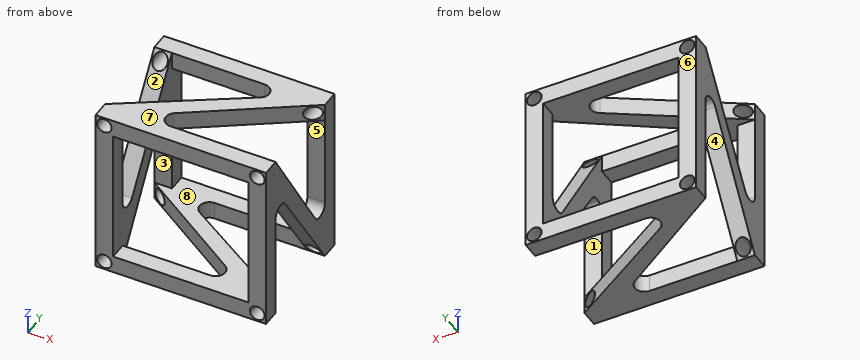
Autodesk Inventor part; units mm, degrees
ref_plane "YZ Plane" through (0, 0, 0) normal (1, 0, 0) x (0, 1, 0)
ref_plane "XZ Plane" through (0, 0, 0) normal (0, 1, 0) x (-1, 0, 0)
ref_plane "XY Plane" through (0, 0, 0) normal (0, 0, 1) x (1, 0, 0)
sketch "Sketch1" plane through (0, 0, 0) normal (0, 1, 0) x (-1, 0, 0)
  line L0 (0, 0) -> (35, 0)
  line L1 (35, 0) -> (35, 35)
  line L2 (35, 35) -> (0, 35)
  line L3 (0, 35) -> (0, 0)
  line L4 (3.6, 3.6) -> (31.4, 3.6)
  line L5 (31.4, 3.6) -> (31.4, 31.4)
  line L6 (31.4, 31.4) -> (3.6, 31.4)
  line L7 (3.6, 31.4) -> (3.6, 3.6)
  circle A0 centre (33.2, 33.2) radius 1.5
  circle A1 centre (33.2, 1.8) radius 1.5
  circle A2 centre (1.8, 1.8) radius 1.5
  circle A3 centre (1.8, 33.2) radius 1.5
  dimension "d0" = 35
  dimension "d1" = 35
  dimension "d2" = 3.6
  dimension "d3" = 3.6
  dimension "d4" = 3.6
  dimension "d5" = 3.6
  dimension "d6" = 3
  dimension "d7" = 1.8
  dimension "d8" = 1.8
  dimension "d9" = 3
  dimension "d10" = 1.8
  dimension "d11" = 1.8
  dimension "d12" = 3
  dimension "d13" = 1.8
  dimension "d14" = 1.8
  dimension "d15" = 3
  dimension "d16" = 1.8
  dimension "d17" = 1.8
extrude "Extrusion1" add sketch "Sketch1" along normal blind 25.9
sketch "Sketch3" plane through (-35, 0, 35) normal (0, 0, 1) x (1, 0, 0)
  line L0 (0, 25.9) -> (35, 25.9)
  line L1 (0, 0) -> (35, 0)
  line L2 (0, 0) -> (0, 25.9)
  line L3 (18.01, 21.1181) -> (18.01, 21.1181)
  line L4 (0, 0) -> (0, 25.9)
  line L5 (31.4, 0) -> (31.4, 25.9)
  line L6 (31.4, 3.6) -> (13.39, 3.6)
  arc A0 (12.1285, 7.1519) -> (13.39, 3.6) centre (13.39, 5.6) ccw
  line L7 (3.6, 22.3) -> (22.6522, 22.3)
  line L8 (3.6, 22.3) -> (0, 22.3)
  line L9 (31.4, 3.6) -> (31.4, 0)
  line L10 (0, 22.3) -> (0, 25.9)
  line L11 (31.4, 22.2467) -> (31.4, 25.9)
  line L12 (0, 3.6) -> (0, 0)
  line L13 (35, 0) -> (35, 25.9)
  line L14 (31.4, 20.2467) -> (31.4, 25.9)
  line L15 (0, 25.9) -> (0, 22.3)
  line L16 (12.1285, 7.1519) -> (35, 22.3)
  arc A1 (23.7216, 18.6099) -> (22.6522, 22.3) centre (22.6522, 20.3) ccw
  line L17 (0, 3.6) -> (23.7216, 18.6099)
  line L18 (3.6, 22.3) -> (3.6, 5.8779)
  line L19 (3.6, 0) -> (3.6, 25.9)
  line L20 (35, 12.95) -> (31.4, 12.95)
  line L21 (3.6, 5.8779) -> (3.6, 12.95)
  line L22 (0, 12.95) -> (0, 3.6)
  line L23 (0, 12.95) -> (3.6, 12.95)
  point P0 (31.4, 19.9157)
  point P1 (0, 22.3)
  dimension "d41" = 18.01
  dimension "d42" = 4
  dimension "d50" = 3.6
  dimension "d67" = 3.6
  dimension "d70" = 3.6
  dimension "d71" = 4
extrude "Extrusion2" cut sketch "Sketch3" against normal blind 3.6 contours L7 A1 L17 L18 | L23 L18 L17 L2 | L13 L20 L5 L16 | L5 L6 A0 L16
sketch "Sketch8" plane through (0, 0, 0) normal (0, 0, -1) x (-1, 0, 0)
  line L0 (0, 25.9) -> (35, 25.9)
  line L1 (0, 0) -> (35, 0)
  line L2 (0, 0) -> (0, 25.9)
  line L3 (18.01, 21.1181) -> (18.01, 21.1181)
  line L4 (0, 0) -> (0, 25.9)
  line L5 (31.4, 0) -> (31.4, 25.9)
  line L6 (31.4, 3.6) -> (13.39, 3.6)
  arc A0 (12.1285, 7.1519) -> (13.39, 3.6) centre (13.39, 5.6) ccw
  line L7 (3.6, 22.3) -> (22.6522, 22.3)
  line L8 (3.6, 22.3) -> (0, 22.3)
  line L9 (31.4, 3.6) -> (31.4, 0)
  line L10 (0, 22.3) -> (0, 25.9)
  line L11 (31.4, 22.2467) -> (31.4, 25.9)
  line L12 (0, 3.6) -> (0, 0)
  line L13 (35, 0) -> (35, 25.9)
  line L14 (31.4, 20.2467) -> (31.4, 25.9)
  line L15 (0, 25.9) -> (0, 22.3)
  line L16 (12.1285, 7.1519) -> (35, 22.3)
  arc A1 (23.7216, 18.6099) -> (22.6522, 22.3) centre (22.6522, 20.3) ccw
  line L17 (0, 3.6) -> (23.7216, 18.6099)
  line L18 (3.6, 22.3) -> (3.6, 5.8779)
  line L19 (3.6, 0) -> (3.6, 25.9)
  line L20 (35, 12.95) -> (31.4, 12.95)
  line L21 (3.6, 5.8779) -> (3.6, 12.95)
  line L22 (0, 12.95) -> (0, 3.6)
  line L23 (0, 12.95) -> (3.6, 12.95)
  point P0 (31.4, 19.9157)
  point P1 (0, 22.3)
  dimension "d80" = 18.01
  dimension "d78" = 4
  dimension "d76" = 3.6
  dimension "d79" = 3.6
  dimension "d77" = 3.6
  dimension "d75" = 4
extrude "Extrusion4" cut sketch "Sketch8" against normal blind 3.6 contours L7 A1 L17 L18 | L23 L18 L17 L2 | L13 L20 L5 L16 | L5 L6 A0 L16
sketch "Sketch9" plane through (0, 0, 35) normal (1, 0, 0) x (0, 0, -1)
  line L0 (0, 25.9) -> (35, 25.9)
  line L1 (0, 0) -> (35, 0)
  line L2 (0, 0) -> (0, 25.9)
  line L3 (18.01, 21.1181) -> (18.01, 21.1181)
  line L4 (0, 0) -> (0, 25.9)
  line L5 (31.4, 0) -> (31.4, 25.9)
  line L6 (31.4, 3.6) -> (13.39, 3.6)
  arc A0 (12.1285, 7.1519) -> (13.39, 3.6) centre (13.39, 5.6) ccw
  line L7 (3.6, 22.3) -> (22.6522, 22.3)
  line L8 (3.6, 22.3) -> (0, 22.3)
  line L9 (31.4, 3.6) -> (31.4, 0)
  line L10 (0, 22.3) -> (0, 25.9)
  line L11 (31.4, 22.2467) -> (31.4, 25.9)
  line L12 (0, 3.6) -> (0, 0)
  line L13 (35, 0) -> (35, 25.9)
  line L14 (31.4, 20.2467) -> (31.4, 25.9)
  line L15 (0, 25.9) -> (0, 22.3)
  line L16 (12.1285, 7.1519) -> (35, 22.3)
  arc A1 (23.7216, 18.6099) -> (22.6522, 22.3) centre (22.6522, 20.3) ccw
  line L17 (0, 3.6) -> (23.7216, 18.6099)
  line L18 (3.6, 22.3) -> (3.6, 5.8779)
  line L19 (3.6, 0) -> (3.6, 25.9)
  line L20 (35, 12.95) -> (31.4, 12.95)
  line L21 (3.6, 5.8779) -> (3.6, 12.95)
  line L22 (0, 12.95) -> (0, 3.6)
  line L23 (0, 12.95) -> (3.6, 12.95)
  point P0 (31.4, 19.9157)
  point P1 (0, 22.3)
  dimension "d89" = 18.01
  dimension "d87" = 4
  dimension "d85" = 3.6
  dimension "d88" = 3.6
  dimension "d86" = 3.6
  dimension "d84" = 4
extrude "Extrusion5" cut sketch "Sketch9" against normal blind 3.6 contours L7 A1 L17 L18 | L23 L18 L17 L2 | L13 L20 L5 L16 | L5 L6 A0 L16
sketch "Sketch10" plane through (-35, 0, 0) normal (-1, 0, 0) x (0, 0, 1)
  line L0 (0, 25.9) -> (35, 25.9)
  line L1 (0, 0) -> (35, 0)
  line L2 (0, 0) -> (0, 25.9)
  line L3 (18.01, 21.1181) -> (18.01, 21.1181)
  line L4 (0, 0) -> (0, 25.9)
  line L5 (31.4, 0) -> (31.4, 25.9)
  line L6 (31.4, 3.6) -> (13.39, 3.6)
  arc A0 (12.1285, 7.1519) -> (13.39, 3.6) centre (13.39, 5.6) ccw
  line L7 (3.6, 22.3) -> (22.6522, 22.3)
  line L8 (3.6, 22.3) -> (0, 22.3)
  line L9 (31.4, 3.6) -> (31.4, 0)
  line L10 (0, 22.3) -> (0, 25.9)
  line L11 (31.4, 22.2467) -> (31.4, 25.9)
  line L12 (0, 3.6) -> (0, 0)
  line L13 (35, 0) -> (35, 25.9)
  line L14 (31.4, 20.2467) -> (31.4, 25.9)
  line L15 (0, 25.9) -> (0, 22.3)
  line L16 (12.1285, 7.1519) -> (35, 22.3)
  arc A1 (23.7216, 18.6099) -> (22.6522, 22.3) centre (22.6522, 20.3) ccw
  line L17 (0, 3.6) -> (23.7216, 18.6099)
  line L18 (3.6, 22.3) -> (3.6, 5.8779)
  line L19 (3.6, 0) -> (3.6, 25.9)
  line L20 (35, 12.95) -> (31.4, 12.95)
  line L21 (3.6, 5.8779) -> (3.6, 12.95)
  line L22 (0, 12.95) -> (0, 3.6)
  line L23 (0, 12.95) -> (3.6, 12.95)
  point P0 (31.4, 19.9157)
  point P1 (0, 22.3)
  dimension "d98" = 18.01
  dimension "d96" = 4
  dimension "d94" = 3.6
  dimension "d97" = 3.6
  dimension "d95" = 3.6
  dimension "d93" = 4
extrude "Extrusion6" cut sketch "Sketch10" against normal blind 3.6 contours L7 A1 L17 L18 | L23 L18 L17 L2 | L13 L20 L5 L16 | L5 L6 A0 L16
properties part number "SolarCar" material "Aluminum 6061"
Here's how the part is built. I have some questions about the finished solid (model axes, mm). Face numbers are marked on the shaded views. A direction names the side the tool comes from. Coordinates: 2 decimals unless noted, no trailing zeros. Write each loop counter-clockwise with the first axis right and the second up, starting at its lowest first coordinate (ties: lowest second). Pieces come first, ordered by that corner, then holes.
Item 1: If we mould it in two halves opening along Z, with no side actions, what happens to the marked faces 5, 6, 7 and 8? For each: +Z half, -Z half, draft (parallel to the pull), parting line (faces both ways), or undercut.
Item 2: I want a section at B-B on z = 8. Write out the boundary of the cut face in (x, y), and give its area (3 significant figures).
Item 3: On a 3-axis mill with a long thin cutter (end or side, diameter ignored), from which of +Z, -Z, +X, -X, +Y, -Y can I reach the whole of each face in a straight line? I mean the marked faces 1, 2, 3 and 4. Say none if no direction works.
Item 4: I want a section at A-A on y = 22.75. Write out the boundary of the cut face in (x, z), and give its area (3 significant figures).
Item 5: Will these pins go through, and if not, where does the flat tip stop? pin 1 (5 mm diameter, centred on x = -33.2, z = 1.8, fed in from -Y); pin 2 (1 mm diameter, centred on y = 10, z = 25, fed in from -X); pin 3 (4 mm diameter, centred on x = -24.5, y = 13.5, fed in from +Z).
Item 6: I want a section at D-D on y = 7.75. Write out the boundary of the cut face in (x, z), and give its area (3 significant figures).
Item 7: I want a section at C-C on x = -15.5. Write out the boundary of the cut face in (y, z).
Item 8: If I drill on line 1 (Z direction, x = -1.8, y = 3.45); line 2 (X direction, y = 3.35, z = 1.8); line 3 (X direction, y = 1.75, z = 8), over which ranges is the centre line in solid material (lowest first)?
Findings below:
1. face 5: undercut
1. face 6: draft
1. face 7: +Z half
1. face 8: undercut
2. outline: (-35, 0) - (-31.4, 0) - (-31.4, 8.66) - (-35, 8.66) - close; (-35, 22.3) - (-31.4, 22.3) - (-31.4, 25.9) - (-35, 25.9) - close; (-3.6, 0) - (0, 0) - (0, 3.6) - (-3.6, 3.6) - close; (-3.6, 17) - (0, 17) - (0, 25.9) - (-3.6, 25.9) - close
2. area: 89.1 mm2
3. face 1: +X
3. face 2: +Z, -X
3. face 3: -X
3. face 4: -Z, -X
4. outline: (-35, 0) - (0, 0) - (0, 35) - (-35, 35) - close; hole circle Ø3 at (-33.2, 1.8); hole circle Ø3 at (-33.2, 33.2); hole (-31.4, 3.6) - (-3.6, 3.6) - (-3.6, 31.4) - (-31.4, 31.4) - close; hole circle Ø3 at (-1.8, 1.8); hole circle Ø3 at (-1.8, 33.2)
4. area: 424 mm2
5. pin 1: stops at y = 0
5. pin 2: stops at x = -3.6
5. pin 3: stops at z = 3.6
6. outline: (-35, 6.56) - (-31.4, 6.56) - (-31.4, 13.03) - (-35, 13.03) - close; (-28.44, 31.4) - (-21.97, 31.4) - (-21.97, 35) - (-28.44, 35) - close; (-13.03, 0) - (-6.56, 0) - (-6.56, 3.6) - (-13.03, 3.6) - close; (-3.6, 21.97) - (0, 21.97) - (0, 28.44) - (-3.6, 28.44) - close
6. area: 93.2 mm2
7. outline: (0, 0) - (3.6, 0) - (3.6, 3.6) - (0, 3.6) - close; (0, 31.4) - (3.6, 31.4) - (3.6, 35) - (0, 35) - close; (9.38, 0) - (13.41, 0) - (13.41, 3.6) - (9.38, 3.6) - close; (12.03, 31.4) - (15.94, 31.4) - (15.94, 35) - (12.03, 35) - close; (22.3, 0) - (25.9, 0) - (25.9, 3.6) - (22.3, 3.6) - close; (22.3, 31.4) - (25.9, 31.4) - (25.9, 35) - (22.3, 35) - close
8. line 1: z = 0 to 0.3, 3.3 to 31.7, 34.7 to 35
8. line 2: x = -35 to -34.7, -31.7 to -3.3, -0.3 to 0
8. line 3: x = -35 to -31.4, -3.6 to 0
